Could you check a few things on this model? Use its own coordinates, in mm. A direction names the side the tool comes from. Round coordinates to 2 decimals unless told otherwise and drop trailing zeros. Write each loop counter-clockwise with the first axis right and the second up, starting at its lowest first coordinate (ties: lowest second). Pieces come first, ordered by that corner, then holes. Notation, with made-up numbers: (36.25, 38.25) -> (82.25, 38.25) arc R14 cw to (82.25, 50.25) -> close; hole circle Ø11 at (44, 84.5). An arc over 180 degrees is marked (long way). Answer in a Markdown table with one row per item.
Autodesk Inventor part; units mm, degrees
ref_plane "YZ Plane" through (0, 0, 0) normal (1, 0, 0) x (0, 1, 0)
ref_plane "XZ Plane" through (0, 0, 0) normal (0, 1, 0) x (-1, 0, 0)
ref_plane "XY Plane" through (0, 0, 0) normal (0, 0, 1) x (1, 0, 0)
sketch "Esboço1" plane through (0, 0, 0) normal (0, 1, 0) x (-1, 0, 0)
  arc A0 (1, 1.118) -> (1, -1.118) centre (0, 0) ccw construction
  line L0 (1, 1.118) -> (1, -1.118) construction
  line L1 (0, 0) -> (-1.5, 0) construction
  line L2 (1.2, -1.2042) -> (1.2, 1.2042)
  arc A1 (1.2, 1.2042) -> (1.2, -1.2042) centre (0, 0) ccw
  circle A2 centre (0, 0) radius 3
  point P0 (1, 0)
  dimension "d0" = 3
  dimension "d1" = 2.5
  dimension "d2" = 0.2
  dimension "d3" = 6
extrude "Extrusão1" add sketch "Esboço1" along normal blind 2
sketch "Esboço2" plane through (0, 2, 0) normal (0, 1, 0) x (1, 0, 0)
  line L0 (0, 0) -> (-5, 0) construction
  line L1 (-5, 0) -> (-5, 0.25)
  line L2 (-5, 0.25) -> (-4.5, 0.5387)
  line L3 (-4.5, 0.5387) -> (-2.8873, 0.5387)
  line L4 (-5, 0) -> (-5, -0.25)
  line L5 (-5, -0.25) -> (-4.5, -0.5387)
  line L6 (-4.5, -0.5387) -> (-2.8873, -0.5387)
  line L7 (-4.3301, -2.5) -> (-4.4551, -2.2835)
  line L8 (-4.4551, -2.2835) -> (-4.1665, -1.7835)
  line L9 (-4.1665, -1.7835) -> (-2.7698, -0.9771)
  line L10 (-4.3301, -2.5) -> (-4.2051, -2.7165)
  line L11 (-4.2051, -2.7165) -> (-3.6278, -2.7165)
  line L12 (-3.6278, -2.7165) -> (-2.2311, -1.9102)
  line L13 (-2.5, -4.3301) -> (-2.7165, -4.2051)
  line L14 (-2.7165, -4.2051) -> (-2.7165, -3.6278)
  line L15 (-2.7165, -3.6278) -> (-1.9102, -2.2311)
  line L16 (-2.5, -4.3301) -> (-2.2835, -4.4551)
  line L17 (-2.2835, -4.4551) -> (-1.7835, -4.1665)
  line L18 (-1.7835, -4.1665) -> (-0.9771, -2.7698)
  line L19 (0, -5) -> (-0.25, -5)
  line L20 (-0.25, -5) -> (-0.5387, -4.5)
  line L21 (-0.5387, -4.5) -> (-0.5387, -2.8873)
  line L22 (0, -5) -> (0.25, -5)
  line L23 (0.25, -5) -> (0.5387, -4.5)
  line L24 (0.5387, -4.5) -> (0.5387, -2.8873)
  line L25 (2.5, -4.3301) -> (2.2835, -4.4551)
  line L26 (2.2835, -4.4551) -> (1.7835, -4.1665)
  line L27 (1.7835, -4.1665) -> (0.9771, -2.7698)
  line L28 (2.5, -4.3301) -> (2.7165, -4.2051)
  line L29 (2.7165, -4.2051) -> (2.7165, -3.6278)
  line L30 (2.7165, -3.6278) -> (1.9102, -2.2311)
  line L31 (4.3301, -2.5) -> (4.2051, -2.7165)
  line L32 (4.2051, -2.7165) -> (3.6278, -2.7165)
  line L33 (3.6278, -2.7165) -> (2.2311, -1.9102)
  line L34 (4.3301, -2.5) -> (4.4551, -2.2835)
  line L35 (4.4551, -2.2835) -> (4.1665, -1.7835)
  line L36 (4.1665, -1.7835) -> (2.7698, -0.9771)
  line L37 (5, 0) -> (5, -0.25)
  line L38 (5, -0.25) -> (4.5, -0.5387)
  line L39 (4.5, -0.5387) -> (2.8873, -0.5387)
  line L40 (5, 0) -> (5, 0.25)
  line L41 (5, 0.25) -> (4.5, 0.5387)
  line L42 (4.5, 0.5387) -> (2.8873, 0.5387)
  line L43 (4.3301, 2.5) -> (4.4551, 2.2835)
  line L44 (4.4551, 2.2835) -> (4.1665, 1.7835)
  line L45 (4.1665, 1.7835) -> (2.7698, 0.9771)
  line L46 (4.3301, 2.5) -> (4.2051, 2.7165)
  line L47 (4.2051, 2.7165) -> (3.6278, 2.7165)
  line L48 (3.6278, 2.7165) -> (2.2311, 1.9102)
  line L49 (2.5, 4.3301) -> (2.7165, 4.2051)
  line L50 (2.7165, 4.2051) -> (2.7165, 3.6278)
  line L51 (2.7165, 3.6278) -> (1.9102, 2.2311)
  line L52 (2.5, 4.3301) -> (2.2835, 4.4551)
  line L53 (2.2835, 4.4551) -> (1.7835, 4.1665)
  line L54 (1.7835, 4.1665) -> (0.9771, 2.7698)
  line L55 (0, 5) -> (0.25, 5)
  line L56 (0.25, 5) -> (0.5387, 4.5)
  line L57 (0.5387, 4.5) -> (0.5387, 2.8873)
  line L58 (0, 5) -> (-0.25, 5)
  line L59 (-0.25, 5) -> (-0.5387, 4.5)
  line L60 (-0.5387, 4.5) -> (-0.5387, 2.8873)
  line L61 (-2.5, 4.3301) -> (-2.2835, 4.4551)
  line L62 (-2.2835, 4.4551) -> (-1.7835, 4.1665)
  line L63 (-1.7835, 4.1665) -> (-0.9771, 2.7698)
  line L64 (-2.5, 4.3301) -> (-2.7165, 4.2051)
  line L65 (-2.7165, 4.2051) -> (-2.7165, 3.6278)
  line L66 (-2.7165, 3.6278) -> (-1.9102, 2.2311)
  line L67 (-4.3301, 2.5) -> (-4.2051, 2.7165)
  line L68 (-4.2051, 2.7165) -> (-3.6278, 2.7165)
  line L69 (-3.6278, 2.7165) -> (-2.2311, 1.9102)
  line L70 (-4.3301, 2.5) -> (-4.4551, 2.2835)
  line L71 (-4.4551, 2.2835) -> (-4.1665, 1.7835)
  line L72 (-4.1665, 1.7835) -> (-2.7698, 0.9771)
  circle A0 centre (0, 0) radius 3
  point P0 (-1.0091, -2.8252)
  point P1 (-1.9421, -2.2865)
  point P2 (-2.2865, -1.9421)
  point P3 (-2.8252, -1.0091)
  point P4 (-2.9512, -0.5387)
  point P5 (-2.9512, 0.5387)
  point P6 (-2.8252, 1.0091)
  point P7 (-2.2865, 1.9421)
  point P8 (-1.9421, 2.2865)
  point P9 (-1.0091, 2.8252)
  point P10 (-0.5387, 2.9512)
  point P11 (0.5387, 2.9512)
  point P12 (1.0091, 2.8252)
  point P13 (1.9421, 2.2865)
  point P14 (2.2865, 1.9421)
  point P15 (2.8252, 1.0091)
  point P16 (2.9512, 0.5387)
  point P17 (2.9512, -0.5387)
  point P18 (2.8252, -1.0091)
  point P19 (2.2865, -1.9421)
  point P20 (1.9421, -2.2865)
  point P21 (1.0091, -2.8252)
  point P22 (0.5387, -2.9512)
  point P23 (-0.5387, -2.9512)
  dimension "d15" = 6
  dimension "d6" = 5
  dimension "d7" = 0.25
  dimension "d9" = 60
  dimension "d10" = 0.5
  dimension "d13" = 360
extrude "Extrusão2" add sketch "Esboço2" against normal blind 2 contours L1 L2 L3 A0 L6 L5 L4 | L72 L71 L70 L67 L68 L69 A0 | A0 L12 L11 L10 L7 L8 L9 | L66 L65 L64 L61 L62 L63 A0 | A0 L18 L17 L16 L13 L14 L15 | L60 L59 L58 L55 L56 L57 A0 | A0 L24 L23 L22 L19 L20 L21 | L54 L53 L52 L49 L50 L51 A0 | A0 L30 L29 L28 L25 L26 L27 | L48 L47 L46 L43 L44 L45 A0 | A0 L36 L35 L34 L31 L32 L33 | L42 L41 L40 L37 L38 L39 A0
properties part number "Gear"
1) For faces 5 (the face through (-3.5, 1, 1.4)), 6 (the face through (2.967, 1.014, 2.335)), 7 (the face through (0.539, 1, -4)), 8 (the face through (0.539, 1, 4)), which set-ups out of +Z, -Z, +X, -X, +Y, -Y let a thin tool reach every point of the face, with its end or its side?
Findings:
| item | result |
|---|---|
| face 5 | -X, +Y, -Y |
| face 6 | +Y, -Y |
| face 7 | -Z, +Y, -Y |
| face 8 | +Z, +Y, -Y |
2) Imagine slicing it at C-C, the plane z = 4. Please give me the cut outline in (x, y).
Findings:
| item | result |
|---|---|
| outline | (-2.72, 0) -> (-1.69, 0) -> (-1.69, 2) -> (-2.72, 2) -> close; (-0.54, 0) -> (0.54, 0) -> (0.54, 2) -> (-0.54, 2) -> close; (1.69, 0) -> (2.72, 0) -> (2.72, 2) -> (1.69, 2) -> close |
3) Imagine slicing it at D-D, the plane x = 3.5. Please give me the cut outline in (y, z), plus the area to 3 significant figures.
Findings:
| item | result |
|---|---|
| outline | (0, -2.64) -> (2, -2.64) -> (2, -1.4) -> (0, -1.4) -> close; (0, -0.54) -> (2, -0.54) -> (2, 0.54) -> (0, 0.54) -> close; (0, 1.4) -> (2, 1.4) -> (2, 2.64) -> (0, 2.64) -> close |
| area | 7.13 mm^2 |
4) Please list where these lines run through material, in increasing order: line 1 (Z direction, x = 0, y = 0.7); line 2 (X direction, y = 1.4, z = 0); line 3 (X direction, y = 1.9, z = -3).
Findings:
| item | result |
|---|---|
| line 1 | z = -5 to -1.7, 1.7 to 5 |
| line 2 | x = -5 to -1.2, 1.7 to 5 |
| line 3 | x = -2.35 to -1.11, -0.54 to 0.54, 1.11 to 2.35 |
5) Thinking about a two-plate mould opening in X: for faces 1 (the face through (0, 2, -2)), 2 (the face through (-2.967, 1.014, -2.335)), 3 (the face through (3.5, 1, 1.4)), 4 (the face through (-3.5, 1, -1.4)), which applies, +X half, -X half, draft (parallel to the pull), parting line (faces both ways), or undercut?
Findings:
| item | result |
|---|---|
| face 1 | draft |
| face 2 | undercut |
| face 3 | +X half |
| face 4 | -X half |
6) Imagine slicing it at B-B, the plane z = 0. Please give me the cut outline in (x, y), plus the area to 3 significant figures.
Findings:
| item | result |
|---|---|
| outline | (-5, 0) -> (-1.2, 0) -> (-1.2, 2) -> (-5, 2) -> close; (1.7, 0) -> (5, 0) -> (5, 2) -> (1.7, 2) -> close |
| area | 14.2 mm^2 |
7) For pin 1 (0.6 mm diameter, centred on x = -4, y = 1, fed in from +Z); pin 2 (0.8 mm diameter, centred on x = -3.5, y = 1, fed in from -Z); pin 3 (0.5 mm diameter, centred on y = 0.5, z = 4, fed in from -X); pin 4 (3 mm diameter, centred on x = 2, z = 0.5, fed in from -Y), each with a flat end and sliding along its axis, tell me the tip position at first contact or that it passes through.
Findings:
| item | result |
|---|---|
| pin 1 | stops at z = 2.72 |
| pin 2 | stops at z = -2.72 |
| pin 3 | stops at x = -2.72 |
| pin 4 | stops at y = 0 |
8) Imagine slicing it at A-A, the plane x = 0. Please give me the cut outline in (y, z).
Findings:
| item | result |
|---|---|
| outline | (0, -5) -> (2, -5) -> (2, -1.7) -> (0, -1.7) -> close; (0, 1.7) -> (2, 1.7) -> (2, 5) -> (0, 5) -> close |
